Here's how the part is built. I have some questions about the finished solid (model axes, mm). A direction names the side the tool comes from. Coordinates: 2 decimals unless noted, no trailing zeros. Order: outer loops, then holes, each group sorted by start corner. A loop starts at its lowest first (then second) coordinate and runs counter-clockwise, first axis right, second up.
```python
from build123d import *


with BuildPart() as part:
    # 草图1 → 旋转1 (revolve)
    with BuildSketch(Plane.XY, mode=Mode.PRIVATE) as revolve_1_sk:
        with BuildLine():
            Line((32.73725094, 12), (35.73725094, 9))
            Line((35.73725094, 9), (35.73725094, 6))
            Line((35.73725094, 6), (35.028753562, 6))
            ThreePointArc((35.028753562, 6), (34.224082532, 6.623318071), (33.346779451, 7.139419019))
            Line((33.346779451, 7.139419019), (33.346779451, 9))
            Line((33.346779451, 9), (17.73725094, 9))
            Line((17.73725094, 9), (17.73725094, 12))
            Line((17.73725094, 12), (32.73725094, 12))
        make_face()
    revolve(revolve_1_sk.sketch.rotate(Axis((0, 0, 0), (1, 0, 0)), 90), axis=Axis((0, 0, 0), (1, 0, 0)))


solid = part.part
```
Q1. If we section it at C-C on x = 21.25: Write out the boundary of the cut face in (y, z), then the cut area to 3 significant figures.
Q2. For faces 1 (the flat face through (35.737, 6, 2)), 2 (the flat face through (33.347, -7, 3)), which set-ups out of +Z, -Z, +X, -X, +Y, -Y let a thin tool reach every point of the face, with its end or its side?
Q3. If we section it at A-A on z = 0: Write out the boundary of the cut face in (x, y), then the cut area to 3 significant figures.
Q4. I need wall thicknesses on L1, parallel to Y at x = 23, z = 0; L2, parallel to Y at x = 33, z = -7; L3, parallel to X at y = -3.5, z = -7.75. Which ranges of each line are inside material? Lowest first, please.
Q5. Will these pins go through, and if not, where does the flat tip stop? pin 1 (2 mm diameter, centred on x = 22.5, y = -2, fed in from -Z); pin 2 (6 mm diameter, centred on x = 32, z = -5.5, fed in from -Y); pin 3 (10 mm diameter, centred on y = 3.5, z = -1.5, fed in from -X); pin 4 (3 mm diameter, centred on x = 30.5, z = -0.5, fed in from +Y).
Q6. We'd pull the mould along Z, two halves only. Please class faces 3 (the cylindrical face through (25.433, -6.083, -6.633)), 4 (the flat face through (17.737, -9, -2)), 5 (the conical face through (35.59, 5.56, -7.26)), 6 (the cylindrical face through (35.378, -1.802, 5.723)): pulls with the +Z half, pulls with the -Z half, needs draft (parallel to the pull), parting line crosses it, or undercut.
Reply:
1. outline: circle Ø24 at (0, 0); hole circle Ø18 at (0, 0)
1. area: 198 mm2
2. face 1: +Z, -Z, +X, +Y, -Y
2. face 2: -X
3. outline: (17.74, -12) - (32.74, -12) - (35.74, -9) - (35.74, -6) - (35.03, -6) arc R8 cw to (33.35, -7.14) - (33.35, -9) - (17.74, -9) - close; (17.74, 9) - (33.35, 9) - (33.35, 7.14) arc R8 cw to (35.03, 6) - (35.74, 6) - (35.74, 9) - (32.74, 12) - (17.74, 12) - close
3. area: 111 mm2
4. L1: y = -12 to -9, 9 to 12
4. L2: y = -9.42 to -5.66, 5.66 to 9.42
4. L3: x = 33.35 to 35.74
5. pin 1: stops at z = -11.96
5. pin 2: stops at y = -11.74
5. pin 3: stops at x = 33.35
5. pin 4: stops at y = 12
6. face 3: undercut
6. face 4: needs draft
6. face 5: parting line crosses it
6. face 6: undercut
